Can you work these out from the model? Positions are in its coordinate system, mm. Round coordinates to 2 decimals unless told otherwise and drop trailing zeros. Answer as a JSON object with one key per item and string values. Group by question number.
1) Please list where these lines run through material, in increasing order: L1, parallel to Z at x = -10.5, y = -60; L2, parallel to Y at x = -10.75, z = 650; L3, parallel to Y at x = -10.4, z = 10. Write a range as [from, to].
2) I'm going to push a flat-ended pin straight in: pin 1 Ø4 at (y, z) = (-16.7, 50) entering from -X. Where does the tip first touch, or does it pass through?
3) Suppose I cut it at A-A, the plane x = -11.75. State how many separate pieces and enclosed holes the cut face has, and give its area (3 significant figures).
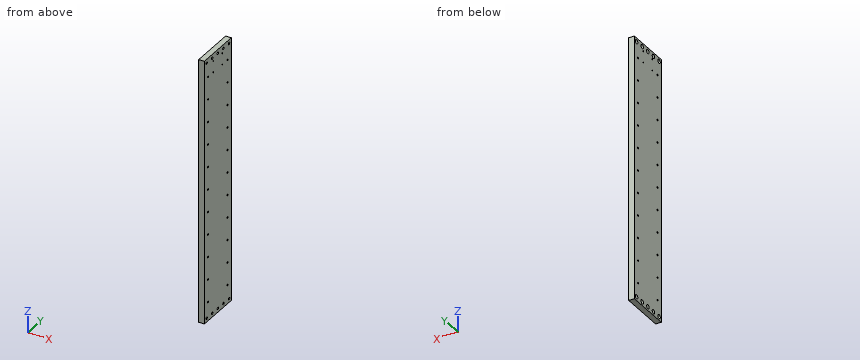
from build123d import *

# Parameters (mm, degrees)
SKETCH2_W                      = 15
SKETCH2_H                      = 120
BOSS_EXTRUDE1_DEPTH            = 700
F_4_5_4_5_DIAMETER_HOLE1_D     = 4.5
M4_TAPPED_HOLE3_D              = 3.3
CBORE_FOR_M6_SHCS1_D           = 6.4
CBORE_FOR_M6_SHCS1_CBORE_D     = 11
CBORE_FOR_M6_SHCS1_CBORE_DEPTH = 6


with BuildPart() as part:
    # Sketch2 → Boss-Extrude1 (new body)
    with BuildSketch(Plane.XY):
        with Locations((-7.5, -60)):
            Rectangle(SKETCH2_W, SKETCH2_H)
    extrude(amount=BOSS_EXTRUDE1_DEPTH)

    # Ø4.5 (4.5) Diameter Hole1 (through all)
    with Locations(Plane(origin=(0, -16.7, 650), x_dir=(0, 0, 1), z_dir=(1, 0, 0))):
        with Locations((0, 0), (-60, 0), (-120, 0), (-180, 0), (-240, 0), (-300, 0), (-360, 0), (-420, 0), (-480, 0), (-540, 0), (-600, 0), (0, 86.6), (-60, 86.6), (-120, 86.6), (-180, 86.6), (-240, 86.6), (-300, 86.6), (-360, 86.6), (-420, 86.6), (-480, 86.6), (-540, 86.6), (-600, 86.6)):
            Hole(F_4_5_4_5_DIAMETER_HOLE1_D / 2)

    # M4 Tapped Hole3 (through all)
    with Locations(Plane(origin=(0, -40, 680), x_dir=(0, 0, 1), z_dir=(1, 0, 0))):
        with Locations((0, 0), (-30, 0), (0, 40), (-30, 40)):
            Hole(M4_TAPPED_HOLE3_D / 2)

    # CBORE for M6 SHCS1 (through all)
    with Locations(Plane(origin=(-15, -10, 690), x_dir=(0, 0, -1), z_dir=(-1, 0, 0))):
        with Locations((0, 0), (0, 50), (0, 25), (0, 75), (0, 100), (680, 0), (680, 25), (680, 50), (680, 75), (680, 100)):
            CounterBoreHole(CBORE_FOR_M6_SHCS1_D / 2, CBORE_FOR_M6_SHCS1_CBORE_D / 2, CBORE_FOR_M6_SHCS1_CBORE_DEPTH)


solid = part.part
Results:
{
 "1": {"L1": "[0, 4.5], [15.5, 684.5], [695.5, 700]", "L2": "[-120, -105.55], [-101.05, -81.65], [-78.35, -41.65], [-38.35, -18.95], [-14.45, 0]", "L3": "[-120, -115.5], [-104.5, -90.5], [-79.5, -65.5], [-54.5, -40.5], [-29.5, -15.5], [-4.5, 0]"},
 "2": {"pin 1": "through"},
 "3": {"separate pieces": "1", "enclosed holes": "36", "area": "82,700 mm^2"}
}
